```python
from build123d import *

# Parameters (mm, degrees)
SKETCH1_R           = 6
BOSS_EXTRUDE1_DEPTH = 8
SKETCH2_R           = 1.55
CUT_EXTRUDE1_DEPTH  = 8


with BuildPart() as part:
    # Sketch1 → Boss-Extrude1 (new body)
    with BuildSketch(Plane(origin=(0, 0, 0), x_dir=(1, 0, 0), z_dir=(0, 1, 0))):
        Circle(SKETCH1_R)
    extrude(amount=BOSS_EXTRUDE1_DEPTH)

    # Sketch2 → Cut-Revolve1 (revolve, cut)
    with BuildSketch(Plane.XY):
        with Locations((6, 3)):
            Circle(SKETCH2_R)
    revolve(axis=Axis((0, 0, 0), (0, 1, 0)), mode=Mode.SUBTRACT)

    # Sketch4 → Cut-Extrude1 (cut)
    with BuildSketch(Plane(origin=(0, 8, 0), x_dir=(1, 0, 0), z_dir=(0, 1, 0))):
        with BuildLine():
            Line((2.367842107, 1.842094434), (-1.105416324, 2.788918537))
            add(Edge.make_bspline(
                [(-1.105416324, 2.788918537), (-1.211764888, 2.742631763), (-1.424454479, 2.650061493), (-1.720250186, 2.465348), (-1.994235491, 2.250550124), (-2.240915768, 2.004518267), (-2.457887126, 1.732083649), (-2.610986563, 1.48525109), (-2.715877402, 1.278481127), (-2.78522539, 1.119080225), (-2.845851316, 0.956099515), (-2.87818707, 0.844775171), (-2.894381942, 0.789020063)],
                knots=[0, 0, 0, 0, 0.124991315, 0.249973772, 0.374969516, 0.499947485, 0.624943228, 0.749921197, 0.812549698, 0.874965023, 0.93737813, 1, 1, 1, 1], degree=3))
            add(Edge.make_bspline(
                [(-2.894381942, 0.789020063), (-2.91771894, 0.693111264), (-2.96416552, 0.502228293), (-2.997819256, 0.209481258), (-3.004051012, -0.084817673), (-2.972979949, -0.476455315), (-2.864367877, -0.958570493), (-2.620857625, -1.498032442), (-2.279511198, -1.981666548), (-1.848081992, -2.386982606), (-1.347643479, -2.703146387), (-0.793946169, -2.912516199), (-0.21061126, -3.013102534), (0.381062278, -2.994642374), (0.958480559, -2.864348225), (1.498072184, -2.620836257), (1.981597519, -2.279616329), (2.29100443, -1.950138678), (2.473270872, -1.700917619), (2.56507701, -1.55952933), (2.648325999, -1.413887775), (2.723092545, -1.264002096), (2.789155439, -1.109821709), (2.84731552, -0.951568689), (2.878651893, -0.84334537), (2.894381942, -0.789020063)],
                knots=[0, 0, 0, 0, 0.031431158, 0.06255602, 0.093680213, 0.125109383, 0.187591007, 0.250067296, 0.312548923, 0.37502521, 0.437506837, 0.499983124, 0.562464749, 0.624941037, 0.687422663, 0.749898951, 0.812380576, 0.874856864, 0.892877316, 0.910755613, 0.928547986, 0.946311478, 0.964103414, 0.981980842, 1, 1, 1, 1], degree=3))
            add(Edge.make_bspline(
                [(2.894381942, -0.789020063), (2.921161696, -0.676169025), (2.974719306, -0.450474947), (3.004425987, -0.103009906), (2.996978881, 0.245057447), (2.94816153, 0.590021165), (2.860396577, 0.9270594), (2.754790092, 1.197638787), (2.652308524, 1.405613669), (2.566396509, 1.55673277), (2.472387401, 1.703022102), (2.402729306, 1.795685419), (2.367842107, 1.842094434)],
                knots=[0, 0, 0, 0, 0.124991314, 0.249973772, 0.374969515, 0.499947485, 0.624943228, 0.749921198, 0.812549697, 0.874965022, 0.937378129, 1, 1, 1, 1], degree=3))
        make_face()
    extrude(amount=-CUT_EXTRUDE1_DEPTH, mode=Mode.SUBTRACT)


solid = part.part
```
Here's how the part is built. I have some questions about the finished solid (model axes, mm). Round coordinates to 2 decimals unless told otherwise and drop trailing zeros. Answer in a Markdown table with one row per item.
Item 1: Thinking about a two-plate mould opening in Z: for faces 1 (the face through (0.656, 4.056, -2.309)), 2 (the face through (0, 8, -3)), 3 (the face through (-6, 1, 0)), which applies, +Z half, -Z half, draft (parallel to the pull), parting line (faces both ways), or undercut?
A:
| item | result |
|---|---|
| face 1 | undercut |
| face 2 | draft |
| face 3 | parting line |
Item 2: If I drill on L1, parallel to X at y = 6, z = -1; L2, parallel to Y at x = 5.25, z = 2.25; L3, parallel to Z at x = 1.5, y = 2.25, over which ranges is the centre line in solid material (lowest first)? Write a range as from..to.
A:
| item | result |
|---|---|
| L1 | x = -5.92..-2.83, 2.83..5.92 |
| L2 | y = 0..1.48, 4.52..8 |
| L3 | z = -4.39..-2.08, 2.6..4.39 |
Item 3: I'm going to push flat-ended pins straight in: pin 1 (1.5 mm diameter, centred on x = -2, y = 5.5, fed in from +Z); pin 2 (4 mm diameter, centred on x = 4, y = 6, fed in from -Z); pin 3 (1 mm diameter, centred on x = 4, y = 6.5, fed in from -Z). Where does each tip first touch, or does it pass through?
A:
| item | result |
|---|---|
| pin 1 | stops at z = 5.87 |
| pin 2 | stops at z = -5.66 |
| pin 3 | stops at z = -4.87 |
